from build123d import *

# Parameters (mm, degrees)
PAD_DEPTH    = 39.8
PAD001_DEPTH = 11
PAD002_DEPTH = 11
PAD003_DEPTH = 6
SKETCH004_R  = 2.5
POCKET_DEPTH = 19.801


with BuildPart() as part:
    # Sketch → Pad (new body)
    with BuildSketch(Plane.XZ):
        Polygon((-23.5, 19.8), (23.5, 19.8), (23.5, 11.3), (16.5, 11.3), (15.5, 0), (7.5, 0), (7.5, 10.8), (-7.5, 10.8), (-7.5, 0), (-15.5, 0), (-16.5, 11.3), (-23.5, 11.3), align=None)
    extrude(amount=PAD_DEPTH)

    # Sketch001 (on Face14 of Pad) → Pad001 (join)
    with BuildSketch(Plane.XZ.offset(39.8)):
        Polygon((-15.5, 0), (-7.5, 0), (-7.5, 10.8), (7.5, 10.8), (7.5, 0), (15.5, 0), (15.5, 19.8), (-15.5, 19.8), align=None)
    extrude(amount=PAD001_DEPTH)

    # Sketch002 (on Face4 of Pad001) → Pad002 (join)
    with BuildSketch(Plane(origin=(0, 0, 0), x_dir=(1, 0, 0), z_dir=(0, 1, 0))):
        Polygon((-15.5, 0), (-7.5, 0), (-7.5, -10.8), (7.5, -10.8), (7.5, 0), (15.5, 0), (15.5, -19.8), (-15.5, -19.8), align=None)
    extrude(amount=PAD002_DEPTH)

    # Sketch003 (on Face19 of Pad002) → Pad003 (join)
    with BuildSketch(Plane.XZ.offset(50.8)):
        Polygon((0, 12.413249), (2.5, 13.856624), (2.5, 16.743376), (0, 18.186751), (-2.5, 16.743376), (-2.5, 13.856624), align=None)
    extrude(amount=PAD003_DEPTH)

    # Sketch004 (on Face1 of Pad003) → Pocket (cut, through all)
    with BuildSketch(Plane(origin=(0, 0, 19.8), x_dir=(-1, 0, 0), z_dir=(0, 0, 1))):
        with Locations((-19, 34.9)):
            Circle(SKETCH004_R)
        with Locations((-19, 4.9)):
            Circle(SKETCH004_R)
        with Locations((19, 4.9)):
            Circle(SKETCH004_R)
        with Locations((19, 34.9)):
            Circle(SKETCH004_R)
    extrude(amount=-POCKET_DEPTH, mode=Mode.SUBTRACT)


solid = part.part
Design review of the part built by this model. Coordinates are the model's own, in mm. A direction names the side the tool comes from. Coordinates: 2 decimals unless noted, no trailing zeros. Loops run counter-clockwise (first coordinate to the right, second up) from the corner with the lowest first, then second, coordinate; pieces in that order, holes last.
Item 1: Add section B-B (z = 15.25). Write out the cut boundary in (x, y), and give its area (3 significant figures).
Completed:
outline: (-23.5, -39.8) - (-15.5, -39.8) - (-15.5, -50.8) - (-2.5, -50.8) - (-2.5, -56.8) - (2.5, -56.8) - (2.5, -50.8) - (15.5, -50.8) - (15.5, -39.8) - (23.5, -39.8) - (23.5, 0) - (15.5, 0) - (15.5, 11) - (-15.5, 11) - (-15.5, 0) - (-23.5, 0) - close; hole circle Ø5 at (-19, -34.9); hole circle Ø5 at (-19, -4.9); hole circle Ø5 at (19, -34.9); hole circle Ø5 at (19, -4.9)
area: 2,500 mm2
Item 2: Wall thickness on L1, parallel to Y at x = 19, z = 16.25; L2, parallel to X at y = -4.9, z = 14.25; L3, parallel to X at y = -50, z = 1: over which ranges is each line inside the solid? List them lowest first.
Completed:
L1: y = -39.8 to -37.4, -32.4 to -7.4, -2.4 to 0
L2: x = -23.5 to -21.5, -16.5 to 16.5, 21.5 to 23.5
L3: x = -15.5 to -7.5, 7.5 to 15.5
Item 3: Add section A-A (x = 19). Write out the cut boundary in (y, z), and give its area (3 significant figures).
Completed:
outline: (-39.8, 11.3) - (-37.4, 11.3) - (-37.4, 19.8) - (-39.8, 19.8) - close; (-32.4, 11.3) - (-7.4, 11.3) - (-7.4, 19.8) - (-32.4, 19.8) - close; (-2.4, 11.3) - (0, 11.3) - (0, 19.8) - (-2.4, 19.8) - close
area: 253 mm2
Item 4: For faces 5 (the flat face through (-1.233, -53.758, 17.475)), 6 (the flat face through (-19, 0, 14)), 7 (the flat face through (-20, -20, 11.3)), 8 (the flat face through (15.5, -45, 10)), list the 3-axis set-ups (+Z, -Z, +X, -X, +Y, -Y) from which the entire face can be reached by the end or side of a thin tool; tool diameter is ignored.
Completed:
face 5: +Z, -X, -Y
face 6: +Z, -Z, -X, +Y
face 7: -Z, -X, +Y, -Y
face 8: +Z, -Z, +X, -Y
Item 5: Clearance check with flat-ended pins moving along their axes: pin 1 (1.4 mm diameter, centred on y = -52.5, z = 15.5, fed in from +X); pin 2 (6.5 mm diameter, centred on x = 19.5, z = 12, fed in from -Y); pin 3 (2 mm diameter, centred on x = -21, y = -26, fed in from -Z); pin 4 (2 mm diameter, centred on x = -13.5, y = -20, fed in from -Z). State where each tip first meets the part, or that it passes through.
Completed:
pin 1: stops at x = 2.5
pin 2: stops at y = -39.8
pin 3: stops at z = 11.3
pin 4: stops at z = 0
Item 6: Draft analysis for pull direction X (two halves, no side actions). For faces 1 (the flat face through (16.007, -19.621, 5.729)), 2 (the flat face through (7.5, -20, 5)), 3 (the flat face through (0, -20, 19.8)), 4 (the flat face through (-1.267, -53.758, 13.145)), state which applies: pulls with the +X half, pulls with the -X half, needs draft (parallel to the pull), parting line crosses it, or undercut.
Completed:
face 1: pulls with the +X half
face 2: undercut
face 3: needs draft
face 4: pulls with the -X half
Item 7: Add section D-D (x = -20). Write out the cut boundary in (y, z), and give its area (3 significant figures).
Completed:
outline: (-39.8, 11.3) - (-37.19, 11.3) - (-37.19, 19.8) - (-39.8, 19.8) - close; (-32.61, 11.3) - (-7.19, 11.3) - (-7.19, 19.8) - (-32.61, 19.8) - close; (-2.61, 11.3) - (0, 11.3) - (0, 19.8) - (-2.61, 19.8) - close
area: 260 mm2
Item 8: Add section C-C (y = 6.5). Write out the cut boundary in (x, z), and give its area (3 significant figures).
Completed:
outline: (-15.5, 0) - (-7.5, 0) - (-7.5, 10.8) - (7.5, 10.8) - (7.5, 0) - (15.5, 0) - (15.5, 19.8) - (-15.5, 19.8) - close
area: 452 mm2
